Autodesk Inventor part; units mm, degrees
sketch "Skizze1" plane through (0, 0, 0) normal (0, 0, 1) x (1, 0, 0)
  line L0 (-15.8, 0) -> (94.8, 0)
  line L1 (0, -28.8) -> (0, 4.8)
  line L2 (0, 0) -> (79, 0)
  line L3 (79, 0) -> (79, -24)
  line L4 (79, -24) -> (0, -24)
  line L5 (0, -24) -> (0, 0)
  dimension "d0" = 79
  dimension "d1" = 24
extrude "Extrusion1" add sketch "Skizze1" along normal blind 5
sketch "Skizze2" plane through (0, 0, 5) normal (0, 0, 1) x (1, 0, 0)
  line L0 (0, -24) -> (79, -24)
  line L1 (0, 0) -> (10, 0)
  line L2 (10, 0) -> (10, -24)
  line L3 (10, -24) -> (0, -24)
  line L4 (0, -24) -> (0, 0)
  dimension "d4" = 10
extrude "Extrusion2" add sketch "Skizze2" along normal blind 35
sketch "Skizze3" plane through (79, -24, 0) normal (1, 0, 0) x (0, 0, -1)
  line L0 (-5, 0) -> (-5, 24)
  line L1 (-5, 10.75) -> (-2, 10.75)
  line L2 (-2, 10.75) -> (-2, 12.75)
  line L3 (-2, 12.75) -> (-5, 12.75)
  line L4 (-5, 12.75) -> (-5, 10.75)
  line L5 (0, 24) -> (-5, 24)
  dimension "d7" = 3
  dimension "d8" = 2
  dimension "d9" = 11.25
extrude "Extrusion3" cut sketch "Skizze3" against normal blind 20
hole "Bohrung1" at (40, -12.25, 5) direction (0, 0, -1) diameter 5 end through all
sketch "Skizze5" plane through (0, -24, 0) normal (-1, 0, 0) x (0, 0, 1)
  line L0 (5, 24) -> (40, 24)
  line L1 (9, 24) -> (9, -0.204)
  line L2 (0, 0) -> (0, 24)
  circle A0 centre (9, 19) radius 2.55
  circle A1 centre (9, 5) radius 2.55
  line L3 (0, 0) -> (40, 0)
  dimension "d26" = 9
  dimension "d27" = 5.1
  dimension "d28" = 5.1
  dimension "d29" = 5
  dimension "d30" = 5
extrude "Extrusion5" cut sketch "Skizze5" against normal blind 30
sketch "Skizze6" plane through (0, 0, 40) normal (0, 0, 1) x (1, 0, 0)
  line L0 (79, -24) -> (0, -24)
  line L1 (0, 0) -> (0, -24)
  line L2 (0, -24) -> (10, -24)
  line L3 (10, -24) -> (10, -13.4534)
  line L4 (10, 0) -> (10, -24)
  line L5 (10, -13.25) -> (2, -13.25)
  line L6 (2, -11.25) -> (10, -11.25)
  line L7 (2, -13.25) -> (2, -11.25)
  line L8 (2, -11.25) -> (10, -11.25)
  line L9 (10, -11.25) -> (10, 0)
  line L10 (0, 0) -> (79, 0)
  line L11 (0, -24) -> (0, 0)
  line L12 (0, 0) -> (0, -24)
  dimension "d33" = 10
sketch "Skizze7" plane through (0, 0, 40) normal (0, 0, 1) x (1, 0, 0)
  line L0 (10, -13.25) -> (2, -13.25)
  line L1 (2, -13.25) -> (10, -13.25)
  point P0 (0, 0)
extrude "Extrusion6" add sketch "Skizze6" along normal blind 15 contours L0 L1 L10 L4 L6 L7 L5 L3
sketch "Skizze8" plane through (0, 0, 55) normal (0, 0, 1) x (1, 0, 0)
  line L0 (10, -11.25) -> (2, -11.25)
  line L1 (2, -13.25) -> (10, -13.25)
  line L2 (2, -11.25) -> (2, -13.25)
  line L3 (2, -13.25) -> (10, -13.25)
  line L4 (10, -13.25) -> (10, -11.25)
  line L5 (10, 0) -> (10, -24)
  line L6 (2, -11.25) -> (10, -11.25)
  point P0 (0, 0)
extrude "Extrusion7" add sketch "Skizze8" against normal blind 35
sketch "Skizze9" plane through (0, 0, 0) normal (0, 1, 0) x (-1, 0, 0)
  point P0 (0, 0)
sketch "Skizze10" plane through (0, 0, 55) normal (0, 0, 1) x (1, 0, 0)
  line L0 (10, 0) -> (10, -24)
  line L1 (10, -13.25) -> (2, -13.25)
  line L2 (2, -13.25) -> (2, -10.75)
  line L3 (2, -10.75) -> (10, -10.75)
  line L4 (10, -10.75) -> (10, -13.25)
  line L5 (10, 0) -> (0, 0)
  line L6 (0, -24) -> (10, -24)
  dimension "d38" = 8
  dimension "d39" = 10.75
  dimension "d40" = 10.75
extrude "Extrusion8" cut sketch "Skizze10" against normal blind 35
properties part number "Gundaufbau"
Could you check a few things on this model? Use its own coordinates, in mm. A direction names the side the tool comes from. Give positions to 0.01 mm unless a question says otherwise; leave off trailing zeros. Write each loop counter-clockwise with the first axis right and the second up, starting at its lowest first coordinate (ties: lowest second). Pieces come first, ordered by that corner, then holes. Notation, with made-up numbers: (17, 87) -> (53, 87) arc R24 ccw to (53, 106) -> close; hole circle Ø8 at (60.5, 81.5). An arc over 180 degrees is marked (long way). Write each question's results on one line, items separated by ' | '. Start each with the question number.
Q1. Suppose I cut it at B-B, the plane x = 40. List the corners of the cut face in (y, z) for me, and give its area (3 significant figures).
Q2. Which directions (+Z, -Z, +X, -X, +Y, -Y) give clear straight access to the entire face, cutting with the end or side of a thin tool? Please do faces 5 (the face through (10, -15, 30)), 6 (the face through (6, -13.25, 38)), 7 (the face through (42.44, -11.71, 2.46)).
Q3. Suppose I cut it at A-A, the plane y = -19. List the corners of the cut face in (x, z) for me, and give its area (3 significant figures).
Q4. I need wall thicknesses on probe 1 along Y at (x, z) = (4, 9); probe 2 along Y at (x, z) = (4.5, 46.5); probe 3 along Z at (x, y) = (7, -19). Which ranges of each line are inside material? Lowest first, please.
Q5. Suppose I cut it at C-C, the plane z = 9. List the corners of the cut face in (x, y) for me.
Q6. We'd pull the mould along Z, two halves only. Please class faces 1 (the face through (4.93, -2.85, 10.37)), 2 (the face through (4.93, -21.26, 10.18)), 3 (the face through (44, -12, 5)), 4 (the face through (0, -12, 27)): +Z half, -Z half, draft (parallel to the pull), parting line (faces both ways), or undercut.
Q7. I'm going to push flat-ended pins straight in: pin 1 Ø2 at (x, y) = (7.5, -12.5) entering from +Z; pin 2 Ø0.8 at (y, z) = (-12.5, 34.5) entering from +X; pin 3 Ø0.6 at (x, y) = (67.5, -12) entering from +Z; pin 4 Ø3 at (x, y) = (63.5, -20) entering from +Z. Where does each tip first touch, or does it pass through?
Q8. Suppose I cut it at D-D, the plane y = -12.25. List the corners of the cut face in (x, z) for me, and give its area (3 significant figures).
Outcome:
1) outline: (-24, 0) -> (-14.75, 0) -> (-14.75, 5) -> (-24, 5) -> close; (-9.75, 0) -> (0, 0) -> (0, 5) -> (-9.75, 5) -> close | area: 95.0 mm2
2) face 5: +Z, +X, +Y, -Y | face 6: +Z, +X | face 7: +Z, -Z
3) outline: (0, 0) -> (79, 0) -> (79, 5) -> (10, 5) -> (10, 6.45) -> (0, 6.45) -> close; (0, 11.55) -> (10, 11.55) -> (10, 55) -> (0, 55) -> close | area: 844 mm2
4) probe 1: -24 to -21.55, -16.45 to -7.55, -2.45 to 0 | probe 2: -24 to -13.25, -10.75 to 0 | probe 3: 0 to 6.45, 11.55 to 55
5) outline: (0, -24) -> (10, -24) -> (10, -21.55) -> (0, -21.55) -> close; (0, -16.45) -> (10, -16.45) -> (10, -7.55) -> (0, -7.55) -> close; (0, -2.45) -> (10, -2.45) -> (10, 0) -> (0, 0) -> close
6) face 1: undercut | face 2: undercut | face 3: +Z half | face 4: draft
7) pin 1: z = 55 | pin 2: x = 2 | pin 3: z = 2 | pin 4: z = 5
8) outline: (0, 0) -> (37.5, 0) -> (37.5, 5) -> (10, 5) -> (10, 20) -> (2, 20) -> (2, 55) -> (0, 55) -> close; (42.5, 0) -> (79, 0) -> (79, 2) -> (59, 2) -> (59, 5) -> (42.5, 5) -> close | area: 530 mm2
